Study the drawing (mm; zero at the part's minimum x, y, z) and answer. A direction names the side the tool comes from. Round coordinates to 2 decimals unless told otherwise and drop trailing zeros. Order: outer loops, then holes, each group sorted by start corner. A loop starts at its lowest first (then second) coordinate and runs counter-clockwise, first axis right, second up. Notation, with made-up numbers: (-25.75, 79.25) - (22.25, 79.25) arc R16 cw to (22.25, 100.25) - close; hole circle Ø11 at (-23, 43). An arc over 180 degrees is marked (long way). Put each result on its own line as item: value. Start each with the question number.
Q1. Section B-B on x = 8.75 is taken. Give the vertices of the cut face in (y, z).
Q2. Section A-A on z = 7.5 is taken. Give the vertices of the cut face in (x, y) (1 decimal).
Q3. Which of the six approach directions +Z, -Z, +X, -X, +Y, -Y give full straight-line access (tool end or side, diameter ignored) to the marked faces 3 and 4?
Q4. Section D-D on y = 62 is taken. Give the vertices of the cut face in (x, z) (1 decimal).
Q5. Find the intervals of material crossed by line 1 along Y through (x, z) = (12.2, 7.5) (1 decimal); line 2 along X through (y, z) = (9, 14); line 3 along Y through (x, z) = (10, 12.5), in increasing order. Write a range as from..to.
Q6. Section C-C on z = 2 is taken. Give the vertices of the cut face in (x, y) (1 decimal).
Q7. Each of these flat-tipped pins is pushed along its axis until it touches: pin 1 Ø6 at (x, y) = (6.5, 49.5) entering from -Z; pin 2 Ø7.5 at (y, z) = (71, 11) entering from -X; pin 3 Ø3 at (y, z) = (56.5, 7.5) entering from -X; pin 4 Ø4 at (x, z) = (7.5, 11.5) entering from +Y. Where does it stop, or does it pass through?
Q8. For a pull along Y with two mould halves and no side action, classify the marked faces 1 and 2 as pulls with the +Y half, pulls with the -Y half, needs draft (parallel to the pull), parting line crosses it, or undercut.
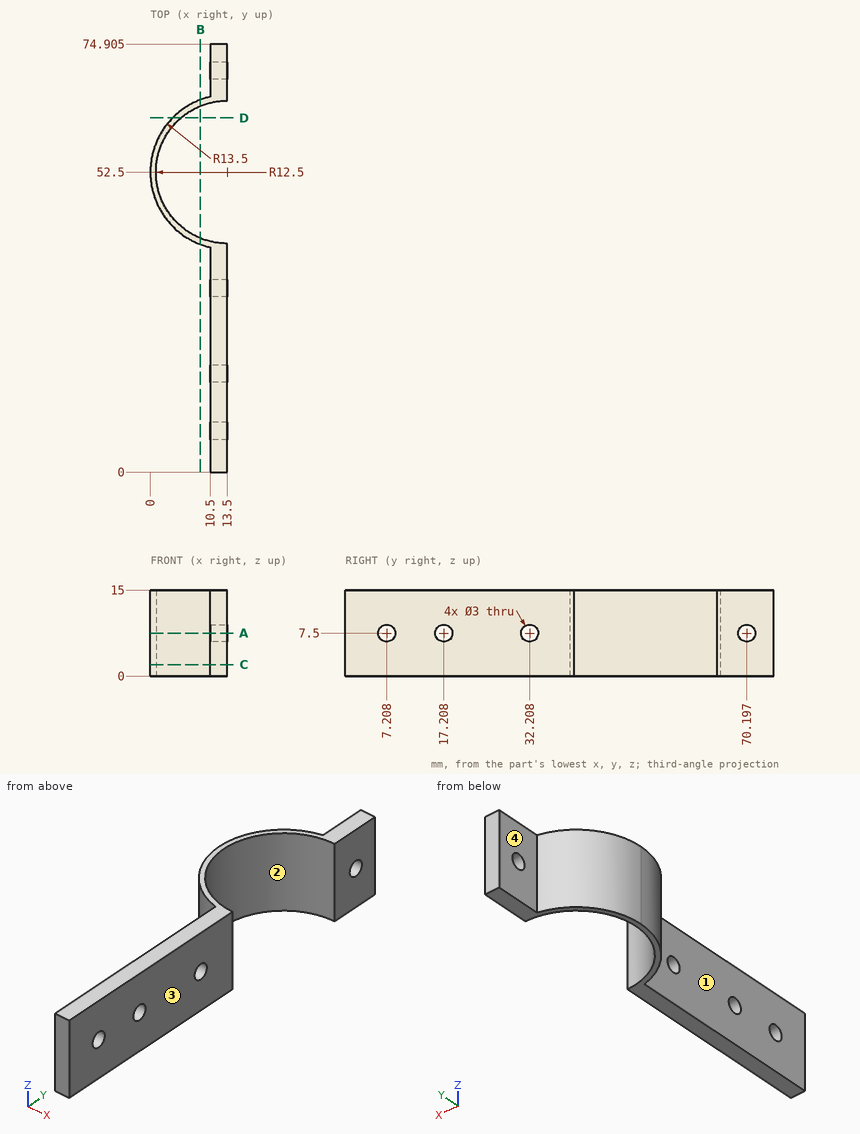
Findings:
1. outline: (39.86, 0) - (40.94, 0) - (40.94, 15) - (39.86, 15) - close; (64.06, 0) - (65.14, 0) - (65.14, 15) - (64.06, 15) - close
2. outline: (10.5, 0) - (13.5, 0) - (13.5, 5.7) - (10.5, 5.7) - close; (10.5, 8.7) - (13.5, 8.7) - (13.5, 15.7) - (10.5, 15.7) - close; (10.5, 18.7) - (13.5, 18.7) - (13.5, 30.7) - (10.5, 30.7) - close; (10.5, 33.7) - (13.5, 33.7) - (13.5, 40) arc R12.5 cw to (13.5, 65) - (13.5, 68.7) - (10.5, 68.7) - (10.5, 65.7) arc R13.5 ccw to (10.5, 39.3) - close; (10.5, 71.7) - (13.5, 71.7) - (13.5, 74.9) - (10.5, 74.9) - close
3. face 3: +Z, -Z, +X, +Y, -Y
3. face 4: +Z, -Z, -X, +Y
4. outline: (3.9, 0) - (5.4, 0) - (5.4, 15) - (3.9, 15) - close
5. line 1: 0..5.7, 8.7..15.7, 18.7..30.7, 33.7..40.1, 64.9..68.7, 71.7..74.9
5. line 2: 10.5..13.5
5. line 3: 39.46..40.5, 64.5..65.54
6. outline: (10.5, 0) - (13.5, 0) - (13.5, 40) arc R12.5 cw to (13.5, 65) - (13.5, 74.9) - (10.5, 74.9) - (10.5, 65.7) arc R13.5 ccw to (10.5, 39.3) - close
7. pin 1: through
7. pin 2: x = 10.5
7. pin 3: x = 0.23
7. pin 4: y = 65.39
8. face 1: needs draft
8. face 2: undercut
